Geometry: final body of the model. Coordinates: model frame, mm. Face numbers are marked on the shaded views. Give positions to 0.01 mm unless a question says otherwise; leave off trailing zeros. Write each loop counter-clockwise with the first axis right and the second up, starting at its lowest first coordinate (ties: lowest second). Pieces come first, ordered by that corner, then holes. Notation, with made-up numbers: (63, 43) - (120, 43) arc R12 cw to (120, 63) - close; hole circle Ø5 at (61.25, 24). An arc over 180 degrees is marked (long way). Return JSON: item names as keys, results as strings.
Autodesk Inventor part; units mm, degrees
ref_plane "YZ Plane" through (0, 0, 0) normal (1, 0, 0) x (0, 1, 0)
ref_plane "XZ Plane" through (0, 0, 0) normal (0, 1, 0) x (-1, 0, 0)
ref_plane "XY Plane" through (0, 0, 0) normal (0, 0, 1) x (1, 0, 0)
sketch "Эскиз1" plane through (0, 0, 0) normal (0, 0, 1) x (1, 0, 0)
  circle A0 centre (4.9, 17.1) radius 0.455
  circle A1 centre (4.9, 17.1) radius 0.7
  line L0 (6.3, 15.875) -> (6.3, 17.1)
  line L1 (0, 21) -> (7, 21)
  line L2 (7, 21) -> (7, 19.75)
  line L3 (7, 19.75) -> (1.75, 19.75)
  line L4 (0, 0) -> (9.5856, 0)
  line L5 (0, 21) -> (0, 17.1)
  line L6 (0, 17.1) -> (1.75, 16.75)
  line L7 (1.75, 16.75) -> (4.9, 15)
  line L8 (4.9, 15) -> (6.3, 15.875)
  line L9 (4.9, 15) -> (0, 15) construction
  line L10 (0, 18) -> (0, -3)
  line L11 (-1.9171, 0) -> (11.5027, 0)
  line L12 (4.2, 17.1) -> (1.75, 17.59)
  line L13 (1.75, 17.59) -> (1.75, 19.75)
  line L14 (6.3, 17.1) -> (5.6, 17.1)
  dimension "d0" = 42
  dimension "d1" = 31.75
  dimension "d2" = 1.25
  dimension "d3" = 0.91
  dimension "d4" = 1.4
  dimension "d5" = 30
  dimension "d6" = 33.5
  dimension "d7" = 34.2
  dimension "d8" = 4.9
  dimension "d9" = 6.3
  dimension "d10" = 7
  dimension "d12" = 1.75
revolve "Базовый элемент" add sketch "Эскиз1" angle 360 about axis through (0, 0, 0) along (1, 0, 0) contours L14 L0 L8 L7 L6 L5 L1 L2 L3 L13 L12 A1
revolve "Пружинные1" add sketch "Эскиз1" angle 360 about axis through (0, 0, 0) along (1, 0, 0) contours A0 | A1
fillet "Сопряжение1" radius 0.4 3 edges at (7, -21, 0) (1.75, -19.75, 0) (0, -21, 0)
equation "\"d0\" = SD2"
equation "\"d1\" = ABDM"
equation "\"d3\" = SPDI"
equation "\"d4\" = SPDA"
equation "\"d5\" = NND"
equation "\"d6\" = TKDM"
equation "\"d7\" = HLDM"
equation "\"d8\" = SPDST"
equation "\"d9\" = SDI"
equation "\"d10\" = SWDT"
equation "\"d12\" = SD"
equation "\"d11\" = RR"
equation "\"SD2\" = 42"
equation "\"SWDT\" = 7"
equation "\"RR\" = 0.4"
equation "\"SD\" = 1.75"
equation "\"NND\" = 30"
equation "\"SPDA\" = 1.4"
equation "\"SPDI\" = 0.91"
equation "\"TKDM\" = 33.5"
equation "\"HLDM\" = 34.2"
equation "\"ABDM\" = 31.75"
equation "\"SDI\" = 6.3"
equation "\"SPDST\" = 4.9"
equation "\"LAB\" = 0.35"
properties part number "Манжет 1-30x42x7 ГОСТ 8752-79" material "Резина"
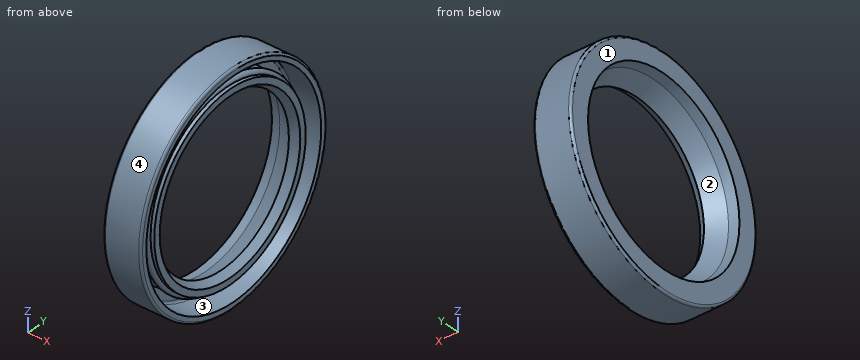
Q1. Section query C-C, the plane x = 3.5. Return the cut outline in (y, z), plus the area to 3 significant figures.
Answer key:
{"outline": "circle Ø42 at (0, 0); circle Ø34.48 at (0, 0); hole circle Ø39.5 at (0, 0); hole circle Ø31.56 at (0, 0)", "area": "312 mm^2"}
Q2. Mould query, pull axis Z, two halves, no side actions, for the marked faces 1, 2, 3 and 4. Classes: pulls with the +Z half, pulls with the -Z half, needs draft (parallel to the pull), parting line crosses it, or undercut.
Answer key:
{"face 1": "needs draft", "face 2": "undercut", "face 3": "undercut", "face 4": "parting line crosses it"}
Q3. Material intervals for probe 1 along Z at (x, y) = (6, 11.5); probe 2 along Z at (x, y) = (6, -2.5); probe 3 along Y at (x, z) = (4, 8.5), sorted ascending. Write a range as [from, to].
Answer key:
{"probe 1": "z = [-17.57, -16.06], [-12.66, -10.67], [10.67, 12.66], [16.06, 17.57]", "probe 2": "z = [-20.85, -19.59], [-16.92, -15.49], [15.49, 16.92], [19.59, 20.85]", "probe 3": "y = [-19.2, -17.83], [-14.88, -12.96], [12.96, 14.88], [17.83, 19.2]"}
Q4. Pin query (flat end, axial travel): P1, Ø2, axis at x = 5.5, z = -5, coming from the +Y side; P2, Ø1, axis at x = 5, y = -4, coming from the +Z side; P3, Ø1, axis at x = 5, y = -1.5, coming from the +Z side. Return the tip coordinate at first contact, or that it passes through.
Answer key:
{"P1": "stops at y = 20.62", "P2": "stops at z = 20.71", "P3": "stops at z = 20.98"}
